The drawing under review shows one solid part. Ordinate dimensions are in mm from its lowest x, y, z. A direction names the side the tool comes from. Give positions to 0.01 mm unless a question says otherwise; leave off trailing zeros. Loops run counter-clockwise (first coordinate to the right, second up) from the corner with the lowest first, then second, coordinate; pieces in that order, holes last. Notation, with made-up numbers: M 10.25,-26 L 14.25,-26 A18 ccw 14.25,0 Z; hole C 39,30 d7. An arc over 180 degrees is marked long. Write item = value, one per line. Start each with the question number.
1. For the marked faces 4 and 5, list the 3-axis set-ups (+Z, -Z, +X, -X, +Y, -Y) from which the entire face can be reached by the end or side of a thin tool; tool diameter is ignored.
2. Draft analysis for pull direction Y (two halves, no side actions). For the marked faces 1, 2 and 3, state which applies: pulls with the +Y half, pulls with the -Y half, needs draft (parallel to the pull), parting line crosses it, or undercut.
3. For pin 1 (8.5 mm diameter, centred on x = 5, y = 67, fed in from -Z); pin 2 (5 mm diameter, centred on y = 55, z = 9.5, fed in from +X); pin 3 (3 mm diameter, centred on y = 15, z = 9.5, fed in from +X), all flat-tipped, find the tip position at first contact; note any pin that passes through.
4. Wall thickness on line 1 along Y through (x, z) = (5, 9.75); line 2 along X through (y, z) = (67, 6.75); line 3 along Y through (x, z) = (35, 1.25): over which ranges is each line inside the solid? List them lowest first. Write a range as from..to.
5. We need section B-B on x = 35. Give the boundary of the cut face in (y, z).
6. We need section C-C on x = 5. Give the boundary of the cut face in (y, z), then the cut area to 3 significant figures.
7. We need section D-D on z = 6.25. Give the boundary of the cut face in (x, y), then the cut area to 3 significant figures.
8. We need section A-A on y = 5. Give the boundary of the cut face in (x, z), then the cut area to 3 significant figures.
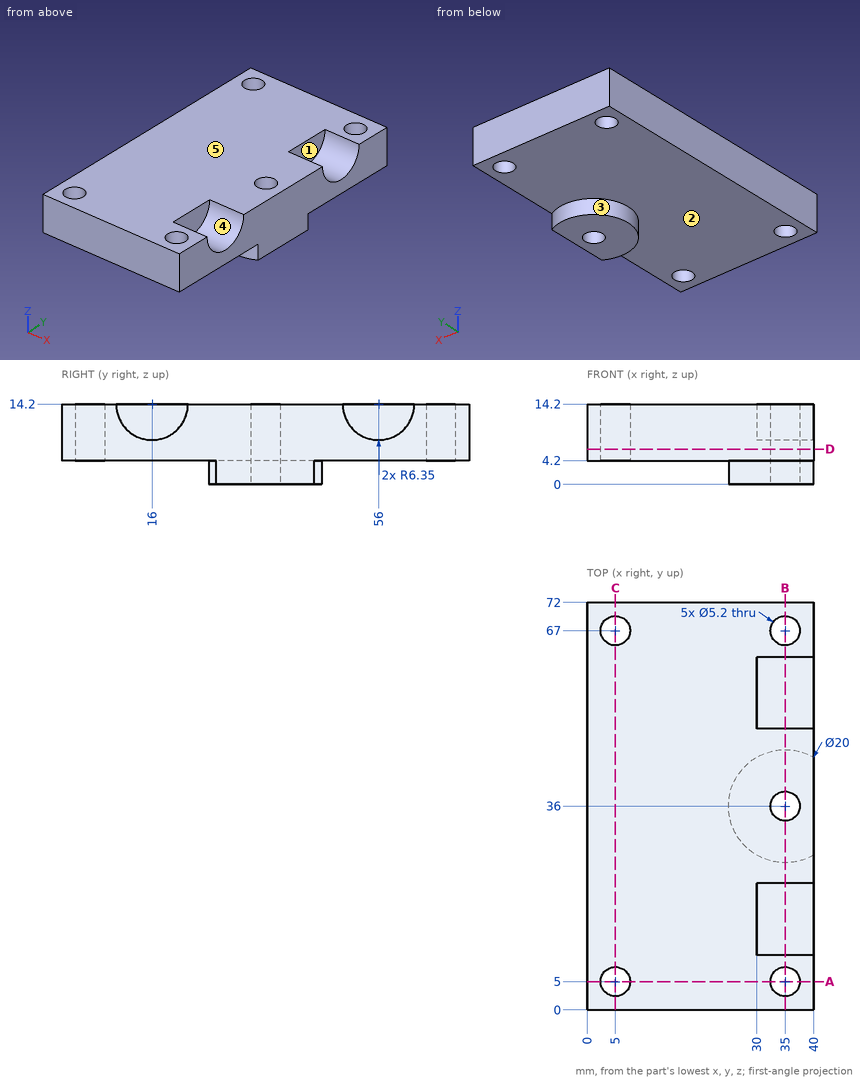
Final values:
q1.face_4 = +Z, +X
q1.face_5 = +Z, +X, -X, +Y, -Y
q2.face_1 = undercut
q2.face_2 = needs draft
q2.face_3 = parting line crosses it
q3.pin_1 = 4.2
q3.pin_2 = 40
q3.pin_3 = 30
q4.line_1 = 0..2.4, 7.6..64.4, 69.6..72
q4.line_2 = 0..2.4, 7.6..32.4, 37.6..40
q4.line_3 = 26..33.4, 38.6..46
q5.outline = M 0,4.2 L 2.4,4.2 L 2.4,14.2 L 0,14.2 Z; M 7.6,4.2 L 26,4.2 L 26,0 L 33.4,0 L 33.4,14.2 L 22.35,14.2 A6.35 cw 9.65,14.2 L 7.6,14.2 Z; M 38.6,0 L 46,0 L 46,4.2 L 64.4,4.2 L 64.4,14.2 L 62.35,14.2 A6.35 cw 49.65,14.2 L 38.6,14.2 Z; M 69.6,4.2 L 72,4.2 L 72,14.2 L 69.6,14.2 Z
q6.outline = M 0,4.2 L 2.4,4.2 L 2.4,14.2 L 0,14.2 Z; M 7.6,4.2 L 64.4,4.2 L 64.4,14.2 L 7.6,14.2 Z; M 69.6,4.2 L 72,4.2 L 72,14.2 L 69.6,14.2 Z
q6.area = 616 mm²
q7.outline = M 0,0 L 40,0 L 40,72 L 0,72 Z; hole C 5,5 d5.2; hole C 5,67 d5.2; hole C 35,5 d5.2; hole C 35,36 d5.2; hole C 35,67 d5.2
q7.area = 2,770 mm²
q8.outline = M 0,4.2 L 2.4,4.2 L 2.4,14.2 L 0,14.2 Z; M 7.6,4.2 L 32.4,4.2 L 32.4,14.2 L 7.6,14.2 Z; M 37.6,4.2 L 40,4.2 L 40,14.2 L 37.6,14.2 Z
q8.area = 296 mm²
